Source: CAD feature listing. Evaluate the final solid. Frame: model axes, mm. Face numbers are marked on the shaded views. A direction names the side the tool comes from. Round coordinates to 2 decimals unless told otherwise and drop trailing zeros. Write each loop counter-clockwise with the first axis right and the second up, starting at its lowest first coordinate (ties: lowest second). Pieces come first, ordered by that corner, then holes.
```python
from build123d import *

# Parameters (mm, degrees)
SKETCH1_W               = 35
SKETCH1_H               = 22.25
BOSS_EXTRUDE1_DEPTH     = 11.5
SKETCH2_R               = 2.2
CUT_EXTRUDE1_DEPTH      = 31.554255023
LPATTERN1_COUNT         = 3
LPATTERN1_PITCH         = 12.7
SKETCH3_W               = 17.5
SKETCH3_H               = 14.50834553
BOSS_EXTRUDE2_DEPTH     = 18
CHAMFER1_SIZE           = 10
BOSS_EXTRUDE3_DEPTH     = 15
BOSS_EXTRUDE4_DEPTH     = 10
CHAMFER2_SIZE           = 7
SKETCH10_R              = 2.35
CUT_EXTRUDE6_DEPTH      = 17
CUT_EXTRUDE7_DEPTH      = 16
CUT_EXTRUDE7_DEPTH_BACK = 4
SKETCH12_R              = 4.2
CHAMFER3_START          = -7.072243188
CHAMFER3_DEPTH          = 22.731839604


with BuildPart() as part:
    # Sketch1 → Boss-Extrude1 (new body)
    with BuildSketch(Plane(origin=(0, 0, 0), x_dir=(0, 0, -1), z_dir=(1, 0, 0))):
        Rectangle(SKETCH1_W, SKETCH1_H)
    extrude(amount=BOSS_EXTRUDE1_DEPTH)

    # Sketch2 → Cut-Extrude1 (cut, through all)
    with BuildSketch(Plane(origin=(0, 11.125, 0), x_dir=(1, 0, 0), z_dir=(0, 1, 0))):
        with Locations(Location((6.35, -10.5, 0), (0, 0, 270))):
            Circle(SKETCH2_R)
    cut_extrude1 = extrude(amount=-CUT_EXTRUDE1_DEPTH, mode=Mode.SUBTRACT)

    # LPattern1: Cut-Extrude1 ×3
    with Locations(*[(0, 0, -i * LPATTERN1_PITCH) for i in range(1, LPATTERN1_COUNT)]):
        add(cut_extrude1, mode=Mode.SUBTRACT)

    # Sketch3 → Boss-Extrude2 (add)
    with BuildSketch(Plane.ZY):
        with Locations((-8.75, -3.870827235)):
            Rectangle(SKETCH3_W, SKETCH3_H)
    extrude(amount=BOSS_EXTRUDE2_DEPTH)

    # Chamfer1
    # the kernel refuses this chamfer: 10 mm, written as the material it adds along each edge
    with BuildSketch(Plane(origin=(0, 3.38334553, 0), x_dir=(0, 0, 1), z_dir=(0, -1, 0))) as chamfer1_piece_1:
        Polygon((CHAMFER1_SIZE, 0), (0, CHAMFER1_SIZE), (0, 0), align=None)
    extrude(amount=14.50834553)
    with BuildSketch(Plane(origin=(0, 3.38334553, -17.5), x_dir=(0, 1, 0), z_dir=(0, 0, 1))) as chamfer1_piece_2_section:
        Polygon((CHAMFER1_SIZE, 0), (0, CHAMFER1_SIZE), (0, 0), align=None)
    chamfer1_piece_2 = extrude(amount=17.5, mode=Mode.PRIVATE)
    chamfer1_piece_2 = split(chamfer1_piece_2, bisect_by=Plane(origin=(0, 11.125, -17.5), z_dir=(0, -1, 0)), keep=Keep.TOP, mode=Mode.PRIVATE)
    add(chamfer1_piece_2)
    with BuildSketch(Plane(origin=(0, 3.38334553, -17.5), x_dir=(0, 1, 0), z_dir=(0, 0, 1))) as chamfer1_piece_3a_section:
        Polygon((CHAMFER1_SIZE, 0), (0, CHAMFER1_SIZE), (0, 0), align=None)
    chamfer1_piece_3a = extrude(amount=43.21682988, mode=Mode.PRIVATE)
    chamfer1_piece_3a = split(chamfer1_piece_3a, bisect_by=Plane(origin=(0, 11.125, -17.5), z_dir=(0, -1, 0)), keep=Keep.TOP, mode=Mode.PRIVATE)
    chamfer1_piece_3a = split(chamfer1_piece_3a, bisect_by=Plane(origin=(0, 3.38334553, 17.5), z_dir=(0, 0, -1)), keep=Keep.TOP, mode=Mode.PRIVATE)
    chamfer1_piece_3a = split(chamfer1_piece_3a, bisect_by=Plane(origin=(0, 3.38334553, 0), z_dir=(0, 0, 1)), keep=Keep.TOP, mode=Mode.PRIVATE)
    with BuildSketch(Plane(origin=(0, 29.100175409, 0), x_dir=(0, 0, 1), z_dir=(0, -1, 0))) as chamfer1_piece_3b_section:
        Polygon((CHAMFER1_SIZE, 0), (0, CHAMFER1_SIZE), (0, 0), align=None)
    chamfer1_piece_3b = extrude(amount=40.225175409, mode=Mode.PRIVATE)
    chamfer1_piece_3b = split(chamfer1_piece_3b, bisect_by=Plane(origin=(0, 11.125, 0), z_dir=(0, -1, 0)), keep=Keep.TOP, mode=Mode.PRIVATE)
    chamfer1_piece_3b = split(chamfer1_piece_3b, bisect_by=Plane(origin=(0, 3.38334553, 0), z_dir=(0, 1, 0)), keep=Keep.TOP, mode=Mode.PRIVATE)
    chamfer1_piece_3 = chamfer1_piece_3a & chamfer1_piece_3b
    add(chamfer1_piece_3)

    # Sketch4 → Boss-Extrude3 (add)
    with BuildSketch(Plane.ZY.offset(18)):
        Polygon((-17.5, -11.125), (-17.5, 3.38334553), (10.639309948, -24.755964418), (-17.5, -24.755964418), (-17.5, -19.755964418), align=None)
    extrude(amount=BOSS_EXTRUDE3_DEPTH)

    # Sketch6 → Boss-Extrude4 (add)
    with BuildSketch(Plane(origin=(-18, 0, 0), x_dir=(0, 0, -1), z_dir=(1, 0, 0))):
        Polygon((17.5, -11.125), (17.5, -24.755964418), (-10.639309948, -24.755964418), (2.99165447, -11.125), align=None)
    extrude(amount=BOSS_EXTRUDE4_DEPTH)

    # Chamfer2
    chamfer2_edges = [part.edges().sort_by_distance(p)[0] for p in [
        (-8, -11.125, -10.245827235),
    ]]
    chamfer(chamfer2_edges, length=CHAMFER2_SIZE)

    # Sketch10 → Cut-Extrude6 (cut)
    with BuildSketch(Plane(origin=(0, -7.058327235, -7.058327235), x_dir=(1, 0, 0), z_dir=(0, 0.7071067811865477, 0.7071067811865475))):
        with Locations(Location((-22.257276658, -13.490437262, 0), (0, 0, 270))):
            Circle(SKETCH10_R)
    extrude(amount=-CUT_EXTRUDE6_DEPTH, mode=Mode.SUBTRACT)

    # Sketch12 → Cut-Extrude7 (cut, two sides: drawn at the far end of the back side and taken through both)
    with BuildSketch(Plane(origin=(0, -23.282012782, -13.732717015), x_dir=(-1, 0, 0), z_dir=(0, -0.8613286818189869, -0.5080481294877154)).offset(-CUT_EXTRUDE7_DEPTH_BACK)):
        with Locations((22.257276658, -6.958686238)):
            Circle(SKETCH12_R)
    extrude(amount=CUT_EXTRUDE7_DEPTH + CUT_EXTRUDE7_DEPTH_BACK, mode=Mode.SUBTRACT)

    # Chamfer3: read off the stored shape, not the designer's step
    # Chamfer3 outline → Chamfer3 (cut)
    with BuildSketch(Plane(origin=(0, 0, 0), x_dir=(1, 0, 0), z_dir=(0, 0.6357072528610996, -0.7719302356170498)).offset(CHAMFER3_START)):
        Polygon((-11, -2.611706712), (-18, 8.195316587), (-18, -4), (-10.100765054, -4), align=None)
    extrude(amount=CHAMFER3_DEPTH, mode=Mode.SUBTRACT)


solid = part.part
```
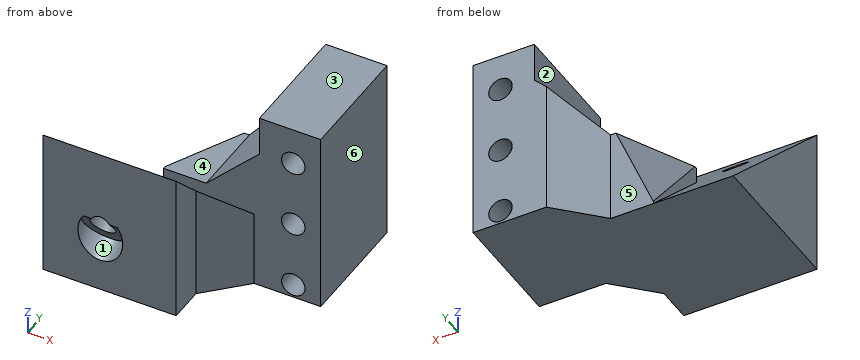
Q1. Set-up query: the marked faces 4, 5 and 6. Return all of +Z, -Z, +X, -X, +Y, -Y with unobstructed straight access to the full face (end or side cutting, diameter ignored); none if empty.
Q2. Section query C-C, the plane z = -14.9. Output: boundary loops of the cut face in (x, y) (3 decimals).
Q3. Line query: line 1 (Z direction, x = 6, y = 0); line 2 (Z direction, x = 7.5, y = -1.5); line 3 (X direction, y = -0.25, z = 10.5). Output: solid intervals per line, ascending.
Q4. Pin query (flat end, axial travel): P1, Ø12, axis at y = 0.5, z = 11.5, coming from the -X side; P2, Ø4, axis at x = -14, y = -4.5, coming from the +Z side; P3, Ø8, axis at y = 1, z = 12.5, coming from the -X side; P4, Ø3.5, axis at x = 6.35, z = -2.2, coming from the -Y side. Return the tip coordinate at first contact, or that it passes through.
Q5. Section query D-D, the plane x = 1. Output: boundary loops of the cut face in (y, z) (3 decimals), and give its area (3 significant figures).
Q6. Section query B-B, the plane y = -8.5. Output: boundary loops of the cut face in (x, z).
Q7. Mould query, pull axis Z, two halves, no side actions, for the marked faces 1, 2 and 3. Classes: pulls with the +Z half, pulls with the -Z half, needs draft (parallel to the pull), parting line crosses it, or undercut.
Q8. Section query A-A, the plane x = 6.35. Output: boundary loops of the cut face in (y, z) (3 decimals).
Filled in:
1. face 4: +Z, -X, +Y
1. face 5: +Z, -Z, -X, +Y
1. face 6: +Z, -Z, +X, +Y, -Y
2. outline: (-33, -24.756) - (-8, -24.756) - (-8, -18.125) - (-1, -11.125) - (4.15, -11.125) - (4.15, 11.125) - (-2.258, 11.125) - (-10, 3.383) - (-17.135, 3.383) - (-18, 1.654) - (-18, 0.783) - (-33, 0.783) - close; (8.55, -11.125) - (11.5, -11.125) - (11.5, 11.125) - (8.55, 11.125) - close
3. line 1: z = -17.5 to -17.07, -12.73 to -4.37, -0.03 to 8.33, 12.67 to 17.5
3. line 2: z = -17.5 to -16.78, -13.02 to -4.08, -0.32 to 8.62, 12.38 to 17.5
3. line 3: x = 0 to 4.15, 8.55 to 11.5
4. P1: stops at x = -4.5
4. P2: stops at z = 0
4. P3: stops at x = -1.5
4. P4: passes through
5. outline: (-11.125, -17.5) - (11.125, -17.5) - (11.125, 17.5) - (-11.125, 17.5) - close
5. area: 779 mm2
6. outline: (-33, -17.5) - (11.5, -17.5) - (11.5, 17.5) - (0, 17.5) - (0, 10) - (-10, 0) - (-16.94, 0) - (-18, -2.57) - (-18, -5.62) - (-33, -5.62) - close; hole circle Ø4.4 at (6.35, -14.9); hole circle Ø4.4 at (6.35, -2.2); hole circle Ø4.4 at (6.35, 10.5)
7. face 1: undercut
7. face 2: needs draft
7. face 3: pulls with the +Z half
8. outline: (-11.125, -17.5) - (11.125, -17.5) - (11.125, -17.1) - (-11.125, -17.1) - close; (-11.125, -12.7) - (11.125, -12.7) - (11.125, -4.4) - (-11.125, -4.4) - close; (-11.125, 0) - (11.125, 0) - (11.125, 8.3) - (-11.125, 8.3) - close; (-11.125, 12.7) - (11.125, 12.7) - (11.125, 17.5) - (-11.125, 17.5) - close
